Could you check a few things on this model? Use its own coordinates, in mm. A direction names the side the tool comes from. Round coordinates to 2 decimals unless told otherwise and drop trailing zeros. Write each loop counter-clockwise with the first axis right and the second up, starting at its lowest first coordinate (ties: lowest second). Pieces come first, ordered by that corner, then holes. Notation, with made-up numbers: (46, 61) -> (67, 61) arc R29 ccw to (67, 87) -> close; hole circle Ø11 at (-8.75, -31.5). An arc over 180 degrees is marked (long way). One line per question, with ' | ' between items. Start each with the question number.
1. Imagine slicing it at C-C, the plane x = 26. List the corners of the cut face in (y, z) for me, and give its area (3 significant figures).
2. Imagine slicing it at D-D, the plane x = 10.5. List the corners of the cut face in (y, z) for me.
3. Imagine slicing it at A-A, the plane z = 5.25. List the corners of the cut face in (x, y) for me.
4. Thinking about a two-plate mould opening in X: for faces 1 (the flat face through (39.471, 153, 0)), 2 (the flat face through (17.558, 146, 5)), 3 (the flat face through (19, 167.892, 4)), which applies, released by +X, released by -X, zero draft, split by the parting line, or undercut?
5. For faces 4 (the flat face through (20.492, 149, 5)), 5 (the flat face through (-0.11, 153, 3)), which set-ups out of +Z, -Z, +X, -X, +Y, -Y let a thin tool reach every point of the face, with its end or its side?
6. For pin 1 Ø3.5 at (x, y) = (9.89, 163.89) entering from +Z; pin 2 Ø8.5 at (x, y) = (19, 155.5) entering from -Z, each with a flat end and sliding along its axis, tell me the tip position at first contact or that it passes through.
7. If I drill on line 1 along X through (y, z) = (148.25, 5.5); line 2 along X through (y, z) = (140, 0.25); line 3 along X through (y, z) = (162.75, 4.75), over which ranges is the centre line in solid material (lowest first)? Write a range as [from, to].
Autodesk Inventor part; units mm, degrees
ref_plane "YZ Plane" through (0, 0, 0) normal (1, 0, 0) x (0, 1, 0)
ref_plane "XZ Plane" through (0, 0, 0) normal (0, 1, 0) x (-1, 0, 0)
ref_plane "XY Plane" through (0, 0, 0) normal (0, 0, 1) x (1, 0, 0)
ref_plane "Work Plane1" through (52.5141, 202.7033, 6.4479) normal (0, 0, -1) x (0, 1, 0)
sketch "Sketch1" plane through (52.5141, 202.7033, 6.4479) normal (0, 0, -1) x (0, 1, 0)
  circle A0 centre (-59.8114, -30.5) radius 1.4 construction
  circle A1 centre (-38.8114, -18.3756) radius 1.4
  circle A2 centre (-38.8114, -42.6244) radius 1.4 construction
  circle A3 centre (41, 0) radius 1.65
  circle A4 centre (-9, 0) radius 1.65
  circle A5 centre (-9, 50) radius 1.65
  circle A6 centre (41, 50) radius 1.65
  circle A7 centre (16, 50) radius 1.65
  circle A8 centre (-9, 25) radius 1.65
  circle A9 centre (16, 0) radius 1.65
  circle A10 centre (41, 25) radius 1.65
  line L0 (80, 55) -> (-80, 55)
  line L1 (-80, 55) -> (-80, -55)
  line L2 (-80, -55) -> (80, -55)
  line L3 (80, -55) -> (80, 55)
  line L4 (-36.5, 0) -> (-36.5, -50)
  line L5 (-14, 0) -> (-36.5, 0)
  line L6 (-14, -5) -> (-14, 0)
  line L7 (72, -5) -> (-14, -5)
  line L8 (72, -50) -> (72, -5)
  line L9 (-36.5, -50) -> (72, -50)
  line L10 (-4, 45) -> (-4, 5)
  line L11 (36, 45) -> (-4, 45)
  line L12 (36, 5) -> (36, 45)
  line L13 (-4, 5) -> (36, 5)
  line L14 (-64.5989, -17.0433) -> (-64.5989, -57.0433) construction
  line L15 (-64.5989, -57.0433) -> (-34.5989, -57.0433) construction
  line L16 (-34.5989, -57.0433) -> (-34.5989, -17.0433) construction
  line L17 (-34.5989, -17.0433) -> (-64.5989, -17.0433) construction
  line L18 (-34.8114, -13.0433) -> (-63.8114, -13.0433)
  line L19 (-63.8114, -13.0433) -> (-63.8114, -52.6244)
  line L20 (-63.8114, -52.6244) -> (-34.8114, -52.6244)
  line L21 (-34.8114, -52.6244) -> (-34.8114, -13.0433)
  circle A11 centre (-59.8114, -30.5) radius 3
  circle A12 centre (-38.8114, -18.3756) radius 3
  circle A13 centre (-38.8114, -42.6244) radius 3 construction
  line L22 (-36.5, -35.1157) -> (-41.75, -35.1157) construction
  line L23 (-41.75, -35.1157) -> (-41.75, -38.5657) construction
  line L24 (-41.75, -38.5657) -> (-56.86, -38.5657) construction
  line L25 (-56.86, -38.5657) -> (-56.86, -35.1157) construction
  line L26 (-56.86, -35.1157) -> (-60.26, -35.1157) construction
  line L27 (-60.26, -35.1157) -> (-60.26, -52.0657) construction
  line L28 (-60.26, -52.0657) -> (-36.5, -52.0657) construction
  line L29 (-36.5, -52.0657) -> (-36.5, -35.1157) construction
  line L30 (-41.75, -28.3657) -> (-36.5, -28.3657) construction
  line L31 (-36.5, -28.3657) -> (-36.5, -25.0657) construction
  line L32 (-36.5, -25.0657) -> (-60.26, -25.0657) construction
  line L33 (-60.26, -25.0657) -> (-60.26, -28.3657) construction
  line L34 (-60.26, -28.3657) -> (-56.86, -28.3657) construction
  line L35 (-56.86, -28.3657) -> (-56.86, -27.0942) construction
  line L36 (-56.86, -27.0942) -> (-41.75, -27.0942) construction
  line L37 (-41.75, -27.0942) -> (-41.75, -28.3657) construction
  line L38 (-56.86, -35.1157) -> (-60.26, -35.1157) construction
  line L39 (-56.86, -38.5657) -> (-56.86, -35.1157) construction
  line L40 (-41.75, -38.5657) -> (-56.86, -38.5657) construction
  line L41 (-41.75, -35.1157) -> (-41.75, -38.5657) construction
  line L42 (-36.5, -35.1157) -> (-41.75, -35.1157) construction
  line L43 (-36.5, -35.05) -> (-36.5, -35.1157) construction
  line L44 (-36.5, -35.05) -> (-56.86, -35.05) construction
  line L45 (-36.5, -34.78) -> (-36.5, -35.05) construction
  line L46 (-36.5, -34.78) -> (-56.86, -34.78) construction
  line L47 (-36.5, -34.51) -> (-36.5, -34.78) construction
  line L48 (-36.5, -34.51) -> (-56.86, -34.51) construction
  line L49 (-36.5, -34.24) -> (-36.5, -34.51) construction
  line L50 (-36.5, -34.24) -> (-56.86, -34.24) construction
  line L51 (-36.5, -33.97) -> (-36.5, -34.24) construction
  line L52 (-36.5, -33.97) -> (-56.86, -33.97) construction
  line L53 (-36.5, -33.7) -> (-36.5, -33.97) construction
  line L54 (-36.5, -33.7) -> (-56.86, -33.7) construction
  line L55 (-36.5, -33.43) -> (-36.5, -33.7) construction
  line L56 (-36.5, -33.43) -> (-56.86, -33.43) construction
  line L57 (-36.5, -33.16) -> (-36.5, -33.43) construction
  line L58 (-36.5, -33.16) -> (-56.86, -33.16) construction
  line L59 (-36.5, -32.89) -> (-36.5, -33.16) construction
  line L60 (-36.5, -32.89) -> (-56.86, -32.89) construction
  line L61 (-36.5, -32.62) -> (-36.5, -32.89) construction
  line L62 (-36.5, -32.62) -> (-56.86, -32.62) construction
  line L63 (-36.5, -32.35) -> (-36.5, -32.62) construction
  line L64 (-36.5, -32.35) -> (-56.86, -32.35) construction
  line L65 (-36.5, -32.08) -> (-36.5, -32.35) construction
  line L66 (-36.5, -32.08) -> (-56.86, -32.08) construction
  line L67 (-36.5, -31.81) -> (-36.5, -32.08) construction
  line L68 (-36.5, -31.81) -> (-56.86, -31.81) construction
  line L69 (-36.5, -31.54) -> (-36.5, -31.81) construction
  line L70 (-36.5, -31.54) -> (-56.86, -31.54) construction
  line L71 (-36.5, -31.27) -> (-36.5, -31.54) construction
  line L72 (-36.5, -31.27) -> (-56.86, -31.27) construction
  line L73 (-36.5, -31) -> (-36.5, -31.27) construction
  line L74 (-36.5, -31) -> (-56.86, -31) construction
  line L75 (-36.5, -30.73) -> (-36.5, -31) construction
  line L76 (-36.5, -30.73) -> (-56.86, -30.73) construction
  line L77 (-36.5, -30.46) -> (-36.5, -30.73) construction
  line L78 (-36.5, -30.46) -> (-56.86, -30.46) construction
  line L79 (-36.5, -30.19) -> (-36.5, -30.46) construction
  line L80 (-36.5, -30.19) -> (-56.86, -30.19) construction
  line L81 (-36.5, -29.92) -> (-36.5, -30.19) construction
  line L82 (-36.5, -29.92) -> (-56.86, -29.92) construction
  line L83 (-36.5, -29.65) -> (-36.5, -29.92) construction
  line L84 (-36.5, -29.65) -> (-56.86, -29.65) construction
  line L85 (-36.5, -29.38) -> (-36.5, -29.65) construction
  line L86 (-36.5, -29.38) -> (-56.86, -29.38) construction
  line L87 (-36.5, -29.11) -> (-36.5, -29.38) construction
  line L88 (-36.5, -29.11) -> (-56.86, -29.11) construction
  line L89 (-36.5, -28.84) -> (-36.5, -29.11) construction
  line L90 (-36.5, -28.84) -> (-56.86, -28.84) construction
  line L91 (-36.5, -28.3657) -> (-36.5, -28.84) construction
  line L92 (-41.75, -28.3657) -> (-36.5, -28.3657) construction
  line L93 (-41.75, -27.0942) -> (-41.75, -28.3657) construction
  line L94 (-56.86, -27.0942) -> (-41.75, -27.0942) construction
  line L95 (-56.86, -28.3657) -> (-56.86, -27.0942) construction
  line L96 (-60.26, -28.3657) -> (-56.86, -28.3657) construction
  line L97 (-60.26, -35.1157) -> (-60.26, -28.3657) construction
  line L98 (-60.26, -25.0657) -> (-36.5, -25.0657) construction
  line L99 (-36.5, -25.0657) -> (-36.5, -52.0657) construction
  line L100 (-60.26, -52.0657) -> (-60.26, -25.0657) construction
  line L101 (-57.1632, -22.5233) -> (-33.4032, -22.5233) construction
  line L102 (-33.4032, -22.5233) -> (-33.4032, -49.5233) construction
  line L103 (-33.4032, -49.5233) -> (-57.1632, -49.5233) construction
  line L104 (-57.1632, -49.5233) -> (-57.1632, -22.5233) construction
  circle A14 centre (-38.8114, -42.6244) radius 3
  point P0 (-202.7033, -52.5141)
  point P1 (-56.7146, -27.9576)
  dimension "d0" = 4
  dimension "d2" = 4
  dimension "d3" = 4
  dimension "d4" = 6
  dimension "d5" = 6
  dimension "d6" = 6
  dimension "d10" = 10
extrude "Extrusion1" add sketch "Sketch1" along normal blind 4 contours L18 L21 L9 L4 A14 A12 | L4 A12 A14 L9 L21 L20 L19 L18
sketch "Sketch2" plane through (52.5141, 202.7033, 2.4479) normal (0, 0, -1) x (-1, 0, 0)
  circle A0 centre (42.6244, -38.8114) radius 3
  circle A1 centre (18.3756, -38.8114) radius 3
  circle A2 centre (30.5, -59.8114) radius 3
  line L0 (13.0433, -34.8114) -> (13.0433, -63.8114)
  line L1 (13.0433, -63.8114) -> (52.6244, -63.8114)
  line L2 (52.6244, -63.8114) -> (52.6244, -34.8114)
  line L3 (52.6244, -34.8114) -> (13.0433, -34.8114)
  point P0 (52.5141, -202.7033)
extrude "Extrusion2" add sketch "Sketch2" along normal blind 1.5 contours A0 | A1 | A2 | L3 L2 L1 L0
sketch "Sketch3" plane through (-0.1103, 138.8919, 6.4479) normal (0, -1, 0) x (1, 0, 0)
  line L0 (39.581, 0) -> (0, 0) construction
  line L1 (0, 0) -> (0, -5.5) construction
  line L2 (39.581, -5.5) -> (0, -5.5)
  line L3 (39.581, 0) -> (39.581, -5.5)
  line L4 (17.5087, -7.4479) -> (17.5087, -6.8479) construction
  line L5 (17.5087, -6.8479) -> (24.2587, -6.8479) construction
  line L6 (24.2587, -6.8479) -> (24.2587, -7.4479) construction
  line L7 (27.5587, -7.4479) -> (24.2587, -7.4479) construction
  line L8 (27.5587, -6.4479) -> (27.5587, -7.4479) construction
  line L9 (27.5587, -6.4479) -> (0.5587, -6.4479) construction
  line L10 (0.5587, -6.4479) -> (0.5587, -7.4479) construction
  line L11 (17.5087, -7.4479) -> (0.5587, -7.4479) construction
  line L12 (39.581, 0) -> (39.581, -5.5) construction
  line L13 (39.581, -5.5) -> (34.1825, -5.5)
  line L14 (34.1825, -5.5) -> (34.1825, -6.25)
  line L15 (34.8694, -6.8) -> (39.581, -6.8)
  line L16 (39.581, -6.8) -> (39.581, -5.5)
  line L17 (39.581, -6.8) -> (32.6714, -6.8)
  line L18 (32.6714, -6.8) -> (34.1825, -6.25)
  line L19 (12.6726, -5.5) -> (12.6726, -6.5)
  line L20 (0, 0) -> (0, -5.5) construction
  line L21 (0, -5.5) -> (2.8846, -5.5)
  line L22 (4.3957, -6.8) -> (0, -6.8)
  line L23 (0, -6.8) -> (0, -5.5)
  line L24 (4.3957, -6.8) -> (4.3957, -6.8)
  line L25 (0, -5.5) -> (39.581, -5.5)
  line L26 (4.3957, -6.8) -> (2.8846, -6.25)
  line L27 (2.8846, -6.25) -> (2.8846, -5.5)
  line L28 (3.4957, -5.5) -> (33.4957, -5.5) construction
  line L29 (33.4957, -5.5) -> (33.4957, -6.5) construction
  line L30 (33.4957, -6.5) -> (3.4957, -6.5) construction
  line L31 (3.4957, -6.5) -> (3.4957, -5.5) construction
  point P0 (8.981, -5.5)
  dimension "d42" = 1.3
  dimension "d43" = 110
  dimension "d45" = 0.75
  dimension "h1" = 0.75
  dimension "d47" = 110
  dimension "d48" = 30
  dimension "d49" = 1
  dimension "d50" = 0.9
  dimension "d51" = 0
extrude "Extrusion3" add sketch "Sketch3" against normal up to surface (29 mm away)
sketch "Sketch6" plane through (52.5141, 202.7033, 6.4479) normal (0, 0, 1) x (1, 0, 0)
  line L0 (-13.0433, -34.8114) -> (-13.0433, -63.8114)
  line L1 (-52.6244, -34.8114) -> (-13.0433, -34.8114)
  line L2 (-52.6244, -63.8114) -> (-52.6244, -34.8114)
  line L3 (-13.0433, -63.8114) -> (-52.6244, -63.8114)
  line L4 (-23.5962, -45.8071) -> (-17.5454, -39.7563)
  line L5 (-17.5454, -39.7563) -> (-19.6668, -37.635)
  line L6 (-19.6668, -37.635) -> (-25.7175, -43.6858)
  line L7 (-25.7175, -43.6858) -> (-23.5962, -45.8071)
  line L8 (-23.5962, -45.8071) -> (-19.6668, -37.635) construction
  line L9 (-17.5454, -39.7563) -> (-25.7175, -43.6858) construction
  line L10 (-39.0797, -45.8071) -> (-43.9064, -40.9803)
  line L11 (-43.9064, -40.9803) -> (-41.7851, -38.859)
  line L12 (-41.7851, -38.859) -> (-36.9583, -43.6858)
  line L13 (-36.9583, -43.6858) -> (-39.0797, -45.8071)
  line L14 (-39.0797, -45.8071) -> (-41.7851, -38.859) construction
  line L15 (-43.9064, -40.9803) -> (-36.9583, -43.6858) construction
  line L16 (-25.7175, -43.6858) -> (-36.9583, -43.6858)
  line L17 (-23.5962, -45.8071) -> (-23.5962, -49.9899)
  line L18 (-23.5962, -49.9899) -> (-39.0797, -49.9899)
  line L19 (-39.0797, -49.9899) -> (-39.0797, -45.8071)
  line L20 (-32.0216, -49.9899) -> (-28.9927, -49.9899)
  line L21 (-28.9927, -49.9899) -> (-28.9927, -57.6065)
  line L22 (-28.9927, -57.6065) -> (-32.0216, -57.6065)
  line L23 (-32.0216, -57.6065) -> (-32.0216, -49.9899)
  line L24 (-39.0797, -45.8071) -> (-39.0797, -49.9899)
  line L25 (-48.2287, -63.8114) -> (-48.2287, -34.8114) construction
  line L26 (-39.0797, -49.9899) -> (-34.9564, -49.9899)
  line L27 (-34.9564, -49.9899) -> (-34.9564, -63.8114)
  line L28 (-34.9564, -63.8114) -> (-39.0797, -63.8114)
  line L29 (-39.0797, -63.8114) -> (-39.0797, -49.9899)
  point P0 (-52.5141, -202.7033)
  point P1 (-21.6315, -41.7211)
  point P2 (-40.4324, -42.333)
  dimension "d35" = 3
  dimension "d36" = 3
  dimension "d37" = 45
  dimension "d38" = 0
extrude "Extrusion6" cut sketch "Sketch6" against normal blind 2 contours L3 L29 L18 L27 | L18 L19 L13 L16 L7 L17 | L18 L21 L22 L23 | L10 L11 L12 L13 | L6 L5 L4 L7
sketch "Sketch7" plane through (-0.1103, 138.8919, 6.4479) normal (0, -1, 0) x (0, 0, 1)
  line L0 (-11.273, -20.7778) -> (-5.5, -20.7778)
  line L1 (-5.5, -20.7778) -> (-5.5, -10.7778)
  line L2 (-5.5, -10.7778) -> (-11.273, -10.7778)
  line L3 (-11.273, -10.7778) -> (-11.273, -20.7778)
  line L4 (-5.5, -34.1825) -> (-5.5, -2.8846)
  point P0 (-6.8, -32.6714)
  dimension "d53" = 10
extrude "Extrusion7" [suppressed]
fillet "Fillet1" [suppressed]
sketch "Sketch8" plane through (-0.1103, 138.8919, 6.4479) normal (0, -1, 0) x (0, 0, 1)
  line L0 (0, 0) -> (-6.8, 0)
  line L1 (0, 0) -> (-6.8, 0)
  circle A0 centre (-7.6471, -15.7336) radius 2.6
  line L2 (-6.8, 0) -> (-6.8, 0)
  point P0 (-6.4479, -0.1103)
  dimension "d58" = 5.2
extrude "Extrusion8" [suppressed]
equation "\"d45\" = h1"
properties part number "cellSTORM_v5_chiptray_old_0"
Geometry results:
1) outline: (138.89, 0.95) -> (167.89, 0.95) -> (167.89, 6.45) -> (159.02, 6.45) -> (159.02, 4.45) -> (152.71, 4.45) -> (152.71, 6.45) -> (138.89, 6.45) -> close | area: 147 mm2
2) outline: (138.89, 0.95) -> (167.89, 0.95) -> (167.89, 6.45) -> (166.83, 6.45) -> (166.83, 2.45) -> (160.95, 2.45) -> (160.95, 4.45) -> (159.83, 4.45) -> (159.83, 6.45) -> (138.89, 6.45) -> close
3) outline: (-0.11, 138.89) -> (13.43, 138.89) -> (13.43, 156.9) -> (9.4, 160.93) arc R3 cw (long way) to (12.37, 162.2) -> (15.56, 159.02) -> (26.8, 159.02) -> (31.18, 163.4) arc R3 cw (long way) to (33.1, 161.08) -> (28.92, 156.9) -> (28.92, 152.71) -> (23.52, 152.71) -> (23.52, 145.49) arc R3 cw (long way) to (20.49, 145.48) -> (20.49, 152.71) -> (17.56, 152.71) -> (17.56, 138.89) -> (39.47, 138.89) -> (39.47, 167.89) -> (-0.11, 167.89) -> close
4) face 1: released by +X | face 2: undercut | face 3: zero draft
5) face 4: +Z | face 5: +Z, -Z, -X, +Y, -Y
6) pin 1: stops at z = 2.45 | pin 2: stops at z = 0.95
7) line 1: x = [-0.11, 13.43], [17.56, 20.49], [23.52, 39.47] | line 2: x = [-0.11, 2.77], [34.07, 39.47] | line 3: x = [-0.11, 7.12], [12.66, 30.53], [36.91, 39.47]
